Design review of the part built by this model. Coordinates are the model's own, in mm. Face numbers are marked on the shaded views. A direction names the side the tool comes from. Coordinates: 2 decimals unless noted, no trailing zeros. Loops run counter-clockwise (first coordinate to the right, second up) from the corner with the lowest first, then second, coordinate; pieces in that order, holes last. Notation, with made-up numbers: M 89.5,46 L 115.5,46 A7 ccw 115.5,57 Z; hole C -23,-20 d2. An arc over 180 degrees is marked long. Answer as CSV lines item,"result". Start each with the question number.
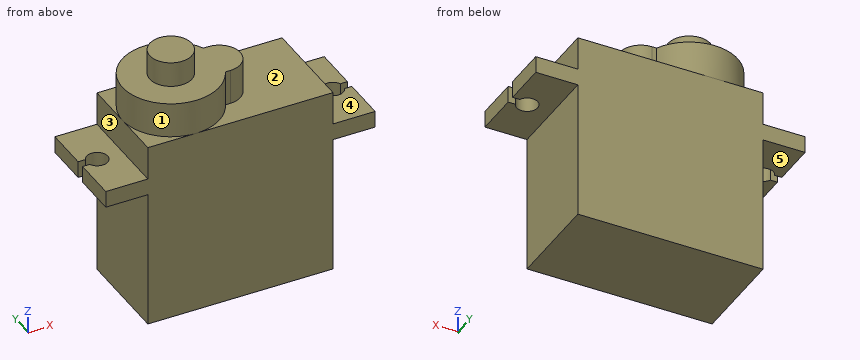
from build123d import *

# Parameters (mm, degrees)
ESQUISSE1_W             = 22
ESQUISSE1_H             = 11.5
BOSS_EXTRU_1_DEPTH      = 22.5
ESQUISSE2_W             = 32
ESQUISSE2_H             = 11.5
BOSS_EXTRU_2_DEPTH      = 2
ENL_V_MAT_EXTRU_1_DEPTH = 35.691497517
BOSS_EXTRU_3_DEPTH      = 4.2
ESQUISSE5_R             = 2.5
BOSS_EXTRU_4_DEPTH      = 3


with BuildPart() as part:
    # Esquisse1 → Boss.-Extru.1 (new body)
    with BuildSketch(Plane.XY):
        with Locations((-11, 5.75)):
            Rectangle(ESQUISSE1_W, ESQUISSE1_H)
    extrude(amount=BOSS_EXTRU_1_DEPTH)

    # Esquisse2 → Boss.-Extru.2 (add)
    with BuildSketch(Plane.XY.offset(18.5)):
        with Locations((-11, 5.75)):
            Rectangle(ESQUISSE2_W, ESQUISSE2_H)
    extrude(amount=-BOSS_EXTRU_2_DEPTH)

    # Esquisse3 → Enl_v. mat.-Extru.1 (cut, through all)
    with BuildSketch(Plane.XY.offset(18.5)):
        with BuildLine():
            Line((4.145643924, 6.25), (5, 6.25))
            Line((5, 6.25), (5, 5.25))
            Line((5, 5.25), (4.145643924, 5.25))
            ThreePointArc((4.145643924, 5.25), (1.75, 5.75), (4.145643924, 6.25))
        make_face()
        with BuildLine():
            Line((-26.145643924, 5.25), (-27, 5.25))
            Line((-27, 5.25), (-27, 6.25))
            Line((-27, 6.25), (-26.145643924, 6.25))
            ThreePointArc((-26.145643924, 6.25), (-23.75, 5.75), (-26.145643924, 5.25))
        make_face()
    extrude(amount=-ENL_V_MAT_EXTRU_1_DEPTH, mode=Mode.SUBTRACT)

    # Esquisse4 → Boss.-Extru.3 (add)
    with BuildSketch(Plane.XY.offset(22.5)):
        with BuildLine():
            Line((-10.5, 8.25), (-11.071921206, 8.25))
            ThreePointArc((-11.071921206, 8.25), (-22, 5.75), (-11.071921206, 3.25))
            Line((-11.071921206, 3.25), (-10.5, 3.25))
            ThreePointArc((-10.5, 3.25), (-8, 5.75), (-10.5, 8.25))
        make_face()
    extrude(amount=BOSS_EXTRU_3_DEPTH)

    # Esquisse5 → Boss.-Extru.4 (add)
    with BuildSketch(Plane.XY.offset(26.7)):
        with Locations(Location((-16.25, 5.75, 0), (0, 0, 180))):
            Circle(ESQUISSE5_R)
    extrude(amount=BOSS_EXTRU_4_DEPTH)


solid = part.part
Item 1: For the marked faces 1, 2, 3, 4 and 5, list the 3-axis set-ups (+Z, -Z, +X, -X, +Y, -Y) from which the entire face can be reached by the end or side of a thin tool; tool diameter is ignored.
Item 2: Add section D-D (x = -15). Give the boundary of the cut face in (y, z).
Item 3: For line 1 along Y through (x, z) = (-25, 17.85); line 2 along Z through (x, y) = (1, 7); line 3 along X through (y, z) = (5.75, 17.2), list the stretches that pass through material, from the lowest coordinate up. Write a range as from..to.
Item 4: Add section C-C (z = 7). Give the boundary of the cut face in (x, y).
Item 5: Add section A-A (x = 3). Give the boundary of the cut face in (y, z).
Item 6: Add section B-B (x = -21). Give the boundary of the cut face in (y, z), plus the area to 3 significant figures.
Item 7: For pin 1 (3.5 mm diameter, centred on x = -7.5, y = 3, fed in from +Z); pin 2 (2 mm diameter, centred on y = 5, z = 5.5, fed in from +X); pin 3 (2 mm diameter, centred on x = 1.5, y = 3, fed in from -Z), all flat-tipped, find the tip position at first contact; note any pin that passes through.
Response:
1,face 1,"+Z"
1,face 2,"+Z, +X"
1,face 3,"+Z, -X, +Y, -Y"
1,face 4,"+Z, +X, +Y, -Y"
1,face 5,"-Z, -X, +Y, -Y"
2,outline,"M 0,0 L 11.5,0 L 11.5,22.5 L 11.36,22.5 L 11.36,26.7 L 7.92,26.7 L 7.92,29.7 L 3.58,29.7 L 3.58,26.7 L 0.14,26.7 L 0.14,22.5 L 0,22.5 Z"
3,line 1,"0..4.5, 7..11.5"
3,line 2,"16.5..18.5"
3,line 3,"-23.75..1.75"
4,outline,"M -22,0 L 0,0 L 0,11.5 L -22,11.5 Z"
5,outline,"M 0,16.5 L 4.5,16.5 L 4.5,18.5 L 0,18.5 Z; M 7,16.5 L 11.5,16.5 L 11.5,18.5 L 7,18.5 Z"
6,outline,"M 0,0 L 11.5,0 L 11.5,22.5 L 8.99,22.5 L 8.99,26.7 L 2.51,26.7 L 2.51,22.5 L 0,22.5 Z"
6,area,"286 mm²"
7,pin 1,"z = 26.7"
7,pin 2,"x = 0"
7,pin 3,"z = 16.5"
